```python
from build123d import *

# Parameters (mm, degrees)
EXTRU_MINCE2_DEPTH       = 200
EPAISSIR5_DEPTH          = 200
EPAISSIR7_DEPTH          = 200
EXTRU_MINCE3_DEPTH       = 20
EXTRU_MINCE3_DEPTH_BACK  = 15
BOSS_EXTRU_2_DEPTH       = 5
ENL_V_MAT_EXTRU_1_DEPTH  = 10
BOSS_EXTRU_3_START       = -212
ESQUISSE12_W             = 35
ESQUISSE12_H             = 45
BOSS_EXTRU_3_DEPTH       = 30
ESQUISSE13_R             = 4
ENL_V_MAT_EXTRU_2_DEPTH  = 250
BOSS_EXTRU_6_DEPTH       = 45
ESQUISSE25_R             = 6
ENL_V_MAT_EXTRU_8_DEPTH  = 45
ENL_V_MAT_EXTRU_9_DEPTH  = 45
ENL_V_MAT_EXTRU_10_DEPTH = 25


# Read off the part's stored shape, not the designer's step: Epaissir5, Epaissir7
with BuildPart() as part:
    # Esquisse3 → Extru.-Mince2 (new body)
    with BuildSketch(Plane.XY):
        with BuildLine():
            Line((-206.649507199, -11.92714811), (-206.649507199, -3.47401752))
            Line((-206.649507199, -3.47401752), (-206.649507199, 81.52598248))
            ThreePointArc((-206.649507199, 81.52598248), (-196.691137759, 105.56761304), (-172.649507199, 115.52598248))
            Line((-172.649507199, 115.52598248), (-82.649507199, 115.52598248))
            ThreePointArc((-82.649507199, 115.52598248), (-58.607876638, 105.56761304), (-48.649507199, 81.52598248))
            Line((-48.649507199, 81.52598248), (-48.649507199, -11.92714811))
            ThreePointArc((-48.649507199, -11.92714811), (-61.399009455, -38.338842544), (-78.173060849, -62.396244951))
            ThreePointArc((-78.173060849, -62.396244951), (-102.275198337, -78.711501116), (-127.649507199, -92.967905467))
            ThreePointArc((-127.649507199, -92.967905467), (-153.023816061, -78.711501116), (-177.125953549, -62.396244951))
            ThreePointArc((-177.125953549, -62.396244951), (-193.900004942, -38.338842544), (-206.649507199, -11.92714811))
        make_face()
        with BuildLine():
            Line((-202.649507199, -11.17401752), (-202.649507199, -3.47401752))
            Line((-202.649507199, -3.47401752), (-202.649507199, 81.52598248))
            ThreePointArc((-202.649507199, 81.52598248), (-193.862710634, 102.739185916), (-172.649507199, 111.52598248))
            Line((-172.649507199, 111.52598248), (-82.649507199, 111.52598248))
            ThreePointArc((-82.649507199, 111.52598248), (-61.436303763, 102.739185916), (-52.649507199, 81.52598248))
            Line((-52.649507199, 81.52598248), (-52.649507199, -11.17401752))
            ThreePointArc((-52.649507199, -11.17401752), (-64.915375774, -36.427970301), (-80.949507199, -59.47401752))
            ThreePointArc((-80.949507199, -59.47401752), (-103.722688687, -74.902894226), (-127.649507199, -88.47401752))
            ThreePointArc((-127.649507199, -88.47401752), (-151.57632571, -74.902894226), (-174.349507199, -59.47401752))
            ThreePointArc((-174.349507199, -59.47401752), (-190.383638623, -36.427970301), (-202.649507199, -11.17401752))
        make_face(mode=Mode.SUBTRACT)
    extrude(amount=EXTRU_MINCE2_DEPTH)

    # Epaissir5 outline → Epaissir5 (add)
    with BuildSketch(Plane.XY):
        with BuildLine():
            add(Edge.make_bspline(
                [(-78.173060849, -62.396244951), (-91.313583381, -75.858349648), (-107.794638855, -86.055391974), (-127.649507199, -92.967905467)],
                knots=[0.501331546, 0.501331546, 0.501331546, 0.501331546, 1, 1, 1, 1], degree=3))
            ThreePointArc((-78.173060849, -62.396244951), (-102.275198337, -78.711501116), (-127.649507199, -92.967905467))
        make_face()
        with BuildLine():
            add(Edge.make_bspline(
                [(-48.649507199, -11.92714811), (-55.127972189, -32.028220402), (-64.962362616, -48.862247174), (-78.173060849, -62.396244951)],
                knots=[0, 0, 0, 0, 0.501331546, 0.501331546, 0.501331546, 0.501331546], degree=3))
            ThreePointArc((-48.649507199, -11.92714811), (-61.399009455, -38.338842545), (-78.173060849, -62.396244951))
        make_face()
    extrude(amount=EPAISSIR5_DEPTH)

    # Epaissir7 outline → Epaissir7 (add)
    with BuildSketch(Plane.XY):
        with BuildLine():
            ThreePointArc((-177.125953549, -62.396244951), (-193.900004942, -38.338842544), (-206.649507199, -11.92714811))
            add(Edge.make_bspline(
                [(-206.649507199, -11.92714811), (-200.171042209, -32.028220402), (-190.336651781, -48.862247174), (-177.125953549, -62.396244951)],
                knots=[0, 0, 0, 0, 0.501331546, 0.501331546, 0.501331546, 0.501331546], degree=3))
        make_face()
        with BuildLine():
            ThreePointArc((-127.649507199, -92.967905467), (-153.023816061, -78.711501116), (-177.125953549, -62.396244951))
            add(Edge.make_bspline(
                [(-177.125953549, -62.396244951), (-163.985431016, -75.858349648), (-147.504375542, -86.055391974), (-127.649507199, -92.967905467)],
                knots=[0.501331546, 0.501331546, 0.501331546, 0.501331546, 1, 1, 1, 1], degree=3))
        make_face()
    extrude(amount=EPAISSIR7_DEPTH)

    # Esquisse7 → Extru.-Mince3 (add, two sides: drawn at the far end of the back side and taken through both)
    with BuildSketch(Plane.XY.offset(200).offset(-EXTRU_MINCE3_DEPTH_BACK)):
        with BuildLine():
            Line((-202.649507199, -11.17401752), (-202.649507199, -3.47401752))
            Line((-202.649507199, -3.47401752), (-202.649507199, 81.52598248))
            ThreePointArc((-202.649507199, 81.52598248), (-193.862710634, 102.739185916), (-172.649507199, 111.52598248))
            Line((-172.649507199, 111.52598248), (-82.649507199, 111.52598248))
            ThreePointArc((-82.649507199, 111.52598248), (-61.436303763, 102.739185916), (-52.649507199, 81.52598248))
            Line((-52.649507199, 81.52598248), (-52.649507199, -11.17401752))
            ThreePointArc((-52.649507199, -11.17401752), (-64.915375774, -36.427970301), (-80.949507199, -59.47401752))
            ThreePointArc((-80.949507199, -59.47401752), (-103.722688687, -74.902894226), (-127.649507199, -88.47401752))
            ThreePointArc((-127.649507199, -88.47401752), (-151.57632571, -74.902894226), (-174.349507199, -59.47401752))
            ThreePointArc((-174.349507199, -59.47401752), (-190.383638623, -36.427970301), (-202.649507199, -11.17401752))
        make_face()
        with BuildLine():
            Line((-200.649507199, -10.794210022), (-200.649507199, -3.47401752))
            Line((-200.649507199, -3.47401752), (-200.649507199, 81.52598248))
            ThreePointArc((-200.649507199, 81.52598248), (-192.448497072, 101.324972353), (-172.649507199, 109.52598248))
            Line((-172.649507199, 109.52598248), (-82.649507199, 109.52598248))
            ThreePointArc((-82.649507199, 109.52598248), (-62.850517326, 101.324972353), (-54.649507199, 81.52598248))
            Line((-54.649507199, 81.52598248), (-54.649507199, -10.794210022))
            ThreePointArc((-54.649507199, -10.794210022), (-66.673062941, -35.471620796), (-82.338728425, -58.013302636))
            ThreePointArc((-82.338728425, -58.013302636), (-104.44621972, -72.997686116), (-127.649507199, -86.221920301))
            ThreePointArc((-127.649507199, -86.221920301), (-150.852794678, -72.997686116), (-172.960285972, -58.013302636))
            ThreePointArc((-172.960285972, -58.013302636), (-188.625951457, -35.471620796), (-200.649507199, -10.794210022))
        make_face(mode=Mode.SUBTRACT)
    extrude(amount=EXTRU_MINCE3_DEPTH + EXTRU_MINCE3_DEPTH_BACK)

    # Esquisse9 → Boss.-Extru.2 (add)
    with BuildSketch(Plane(origin=(0, 0, 0), x_dir=(-1, 0, 0), z_dir=(0, 0, -1))):
        with BuildLine():
            Line((172.649507199, 111.52598248), (82.649507199, 111.52598248))
            ThreePointArc((82.649507199, 111.52598248), (61.436303763, 102.739185916), (52.649507199, 81.52598248))
            Line((52.649507199, 81.52598248), (52.649507199, -11.17401752))
            ThreePointArc((52.649507199, -11.17401752), (79.415793498, -60.238358109), (127.649507199, -88.47401752))
            ThreePointArc((127.649507199, -88.47401752), (175.815578629, -60.172728481), (202.649507199, -11.17401752))
            Line((202.649507199, -11.17401752), (202.649507199, 81.52598248))
            ThreePointArc((202.649507199, 81.52598248), (193.862710634, 102.739185916), (172.649507199, 111.52598248))
        make_face()
    extrude(amount=-BOSS_EXTRU_2_DEPTH)

    # Esquisse10 → Enlèv. mat.-Extru.1 (cut)
    with BuildSketch(Plane(origin=(0, 115.52598248, 0), x_dir=(1, 0, 0), z_dir=(0, 1, 0))):
        with BuildLine():
            Line((-127.649507199, -100), (-120.149507199, -100))
            ThreePointArc((-120.149507199, -100), (-113.078439387, -102.928932188), (-110.149507199, -110))
            Line((-110.149507199, -110), (-110.149507199, -135))
            ThreePointArc((-110.149507199, -135), (-113.078439387, -142.071067812), (-120.149507199, -145))
            Line((-120.149507199, -145), (-135.149507199, -145))
            ThreePointArc((-135.149507199, -145), (-142.220575011, -142.071067812), (-145.149507199, -135))
            Line((-145.149507199, -135), (-145.149507199, -110))
            ThreePointArc((-145.149507199, -110), (-142.220575011, -102.928932188), (-135.149507199, -100))
            Line((-135.149507199, -100), (-127.649507199, -100))
        make_face()
    extrude(amount=-ENL_V_MAT_EXTRU_1_DEPTH, mode=Mode.SUBTRACT)

    # Esquisse12 → Boss.-Extru.3 (add)
    with BuildSketch(Plane(origin=(0, 115.52598248, 0), x_dir=(1, 0, 0), z_dir=(0, 1, 0)).offset(BOSS_EXTRU_3_START)):
        with Locations((-127.649507199, -122.5)):
            Rectangle(ESQUISSE12_W, ESQUISSE12_H)
    extrude(amount=BOSS_EXTRU_3_DEPTH)

    # Esquisse13 → Enlèv. mat.-Extru.2 (cut)
    with BuildSketch(Plane(origin=(0, 115.52598248, 0), x_dir=(1, 0, 0), z_dir=(0, 1, 0))):
        with Locations(Location((-120.149507199, -107.5, 0), (0, 0, 180))):
            Circle(ESQUISSE13_R)
        with Locations(Location((-135.149507199, -107.5, 0), (0, 0, 180))):
            Circle(ESQUISSE13_R)
        with Locations(Location((-135.149507199, -137.5, 0), (0, 0, 180))):
            Circle(ESQUISSE13_R)
        with Locations(Location((-120.149507199, -137.5, 0), (0, 0, 180))):
            Circle(ESQUISSE13_R)
    extrude(amount=-ENL_V_MAT_EXTRU_2_DEPTH, mode=Mode.SUBTRACT)

    # Esquisse23 → Boss.-Extru.6 (add)
    with BuildSketch(Plane(origin=(0, 115.52598248, 0), x_dir=(1, 0, 0), z_dir=(0, 1, 0))):
        Polygon((-172.649507199, 0), (-172.649507199, -30), (-206.649507199, -30), (-246.649507199, -30), (-246.649507199, 0), align=None)
    extrude(amount=-BOSS_EXTRU_6_DEPTH)

    # Esquisse25 → Enlèv. mat.-Extru.8 (cut)
    with BuildSketch(Plane(origin=(0, 115.52598248, 0), x_dir=(1, 0, 0), z_dir=(0, 1, 0))):
        with Locations(Location((-226.649507199, -15, 0), (0, 0, 180))):
            Circle(ESQUISSE25_R)
    extrude(amount=-ENL_V_MAT_EXTRU_8_DEPTH, mode=Mode.SUBTRACT)

    # Esquisse26 → Enlèv. mat.-Extru.9 (cut)
    with BuildSketch(Plane(origin=(0, 115.52598248, 0), x_dir=(1, 0, 0), z_dir=(0, 1, 0))):
        with BuildLine():
            Line((-246.649507199, 0), (-246.649507199, -8))
            ThreePointArc((-246.649507199, -8), (-244.306361448, -2.343145751), (-238.649507199, 0))
            Line((-238.649507199, 0), (-246.649507199, 0))
        make_face()
        with BuildLine():
            ThreePointArc((-238.649507199, -30), (-244.306361448, -27.656854249), (-246.649507199, -22))
            Line((-246.649507199, -22), (-246.649507199, -30))
            Line((-246.649507199, -30), (-238.649507199, -30))
        make_face()
    extrude(amount=-ENL_V_MAT_EXTRU_9_DEPTH, mode=Mode.SUBTRACT)

    # Esquisse27 → Enlèv. mat.-Extru.10 (cut)
    with BuildSketch(Plane.XY.offset(30)):
        with BuildLine():
            Line((-172.649507199, 70.52598248), (-172.649507199, 90.52598248))
            ThreePointArc((-172.649507199, 90.52598248), (-178.507371575, 76.383846856), (-192.649507199, 70.52598248))
            Line((-192.649507199, 70.52598248), (-172.649507199, 70.52598248))
        make_face()
    extrude(amount=-ENL_V_MAT_EXTRU_10_DEPTH, mode=Mode.SUBTRACT)


solid = part.part
```
The listing builds one solid part. Answer for the finished solid, in the listing's coordinates (mm). A direction names the side the tool comes from. Give positions to 0.01 mm unless a question says otherwise; leave off trailing zeros. Order: outer loops, then holes, each group sorted by start corner. A loop starts at its lowest first (then second) coordinate and runs counter-clockwise, first axis right, second up. Notation, with made-up numbers: (6, 21) - (15, 21) arc R20 cw to (15, 41) - close; hole circle Ø3 at (16, 85.25). An arc over 180 degrees is marked (long way). Use one line per item in the form item = value. Start each with the question number.
(1) Flat-ended cylindrical pins translate along their axes: pin 1 Ø1 at (x, z) = (-144, 123) entering from +Y; pin 2 Ø12 at (x, z) = (-164.5, 43) entering from -Y; pin 3 Ø1 at (x, y) = (-160, 14.5) entering from +Z. Find the tip coordinate at first contact, or state that the pin passes through.
(2) A cutting plane is placed at A-A, the plane z = 206. Write down the section's boundary in (x, y).
(3) Consider line 1 (X direction, y = 48, z = 98); line 2 (Z direction, x = -173, y = 20); line 3 (X direction, y = -31, z = 106.5). Determine where each line is inside the solid, lowest interval first. Write a range as from..to.
(4) The mould has two halves that part along X. Classify faces 1 (the cylindrical face through (-142.3, 113.55, 103.01)), 2 (the flat face through (-128, -94, 100)), 3 (the cylindrical face through (-196.954, 105.302, 113.81)): released by +X, released by -X, zero draft, split by the parting line, or undercut.
(5) For faces 4 (the cylindrical face through (-151.249, -75.106, 209.86)), 5 (the flat face through (-128, -94, 145)), 6 (the cylindrical face through (-61.7, 103, 209.9)), determine the directions among +Z, -Z, +X, -X, +Y, -Y from which every point of the face is accessible in a straight line to the end or side of a thin tool.
(6) A cutting plane is placed at B-B, the plane y = 62. Write down the section's boundary in (x, z).
(7) A cutting plane is placed at C-C, the plane z = 15. State how many separate pieces and enclosed holes the cut face has, then the cut area to 3 significant figures.
Ans:
q1.pin_1 = -66.47
q1.pin_2 = -77.83
q1.pin_3 = 5
q2.outline = (-202.65, -11.17) arc R180.47 ccw to (-174.35, -59.47) arc R346.01 ccw to (-127.65, -88.47) arc R346.01 ccw to (-80.95, -59.47) arc R180.47 ccw to (-52.65, -11.17) - (-52.65, 81.53) arc R30 ccw to (-82.65, 111.53) - (-172.65, 111.53) arc R30 ccw to (-202.65, 81.53) - close; hole (-200.65, -10.79) arc R178.47 ccw to (-172.96, -58.01) arc R344.01 ccw to (-127.65, -86.22) arc R344.01 ccw to (-82.34, -58.01) arc R178.47 ccw to (-54.65, -10.79) - (-54.65, 81.53) arc R28 ccw to (-82.65, 109.53) - (-172.65, 109.53) arc R28 ccw to (-200.65, 81.53) - close
q3.line_1 = -206.65..-202.65, -52.65..-48.65
q3.line_2 = 0..5
q3.line_3 = -199.02..-193.44, -61.86..-56.28
q4.face_1 = undercut
q4.face_2 = zero draft
q4.face_3 = released by -X
q5.face_4 = +Z, -X, -Y
q5.face_5 = +Z, -Y
q5.face_6 = +Z, +X, +Y
q6.outline = (-206.65, 0) - (-48.65, 0) - (-48.65, 200) - (-52.65, 200) - (-52.65, 220) - (-54.65, 220) - (-54.65, 185) - (-52.65, 185) - (-52.65, 5) - (-202.65, 5) - (-202.65, 185) - (-200.65, 185) - (-200.65, 220) - (-202.65, 220) - (-202.65, 200) - (-206.65, 200) - close
q7.separate_pieces = 2
q7.enclosed_holes = 1
q7.area = 5,130 mm^2
